Build history of the part. All positions in model axes, mm. Face numbers are marked on the shaded views. A direction names the side the tool comes from. Round coordinates to 2 decimals unless told otherwise and drop trailing zeros. Loops run counter-clockwise (first coordinate to the right, second up) from the corner with the lowest first, then second, coordinate; pieces in that order, holes last. Notation, with made-up numbers: (20.25, 11.5) - (76.25, 11.5) arc R24 ccw to (76.25, 43.5) - close; hole circle Ø10 at (24.5, 80.25). An arc over 180 degrees is marked (long way). Answer as CSV lines item,"result". Start each with the question number.
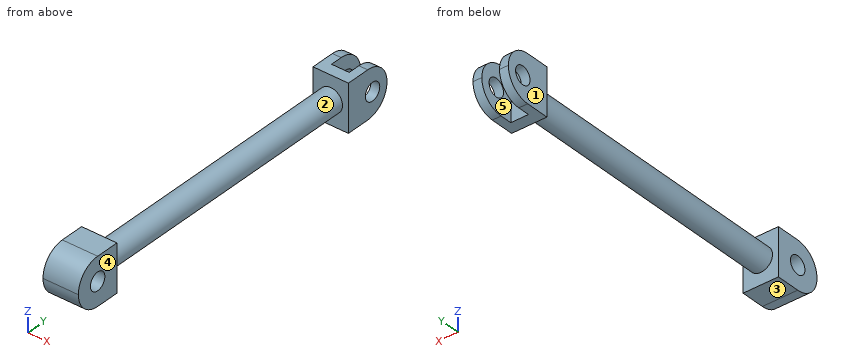
```python
from build123d import *

# Parameters (mm, degrees)
F0_R      = 12.7
F1_DEPTH  = 304.8
F2_W      = 38.1
F2_H      = 50.8
F3_DEPTH  = 50.8
F4_R      = 9.525
F5_DEPTH  = 38.101
F6_W      = 38.1
F6_H      = 50.8
F7_DEPTH  = 50.8
F8_W      = 19.05
F8_H      = 50.8
F9_DEPTH  = 38.1
F10_R     = 9.525
F11_DEPTH = 38.101
F12_R     = 25.39999


# Not quite as in the source:
# - a fillet or chamfer is up to 0.001 mm smaller than in the source, because OpenCascade refuses the exact size


with BuildPart() as f1:
    # F0 (on Front) → F1 (new body)
    with BuildSketch(Plane.XZ):
        Circle(F0_R)
    extrude(amount=F1_DEPTH)

    # F2 (on face) → F3 (join)
    with BuildSketch(Plane.XZ.offset(304.8)):
        Rectangle(F2_W, F2_H)
    extrude(amount=F3_DEPTH)

    # F4 (on face) → F5 (cut, through all)
    with BuildSketch(Plane(origin=(-19.05, 0, 0), x_dir=(0, -1, 0), z_dir=(-1, 0, 0))):
        with Locations((330.2, 0)):
            Circle(F4_R)
    extrude(amount=-F5_DEPTH, mode=Mode.SUBTRACT)

    # F6 (on face) → F7 (join)
    with BuildSketch(Plane(origin=(0, 0, 0), x_dir=(-1, 0, 0), z_dir=(0, 1, 0))):
        Rectangle(F6_W, F6_H)
    extrude(amount=F7_DEPTH)

    # F8 (on face) → F9 (cut)
    with BuildSketch(Plane(origin=(0, 50.8, 0), x_dir=(-1, 0, 0), z_dir=(0, 1, 0))):
        Rectangle(F8_W, F8_H)
    extrude(amount=-F9_DEPTH, mode=Mode.SUBTRACT)

    # F10 (on face) → F11 (cut, through all)
    with BuildSketch(Plane.YZ.offset(19.05)):
        with Locations((31.75, 0)):
            Circle(F10_R)
    extrude(amount=-F11_DEPTH, mode=Mode.SUBTRACT)

    # F12 (radius 25.4 in the source; OpenCascade refuses exactly that, so slightly less here)
    f12_edges = [f1.edges().sort_by_distance(p)[0] for p in [
        (14.2875, 50.8, 25.4),
        (14.2875, 50.8, -25.4),
        (-14.2875, 50.8, -25.4),
        (-14.2875, 50.8, 25.4),
        (0, -355.6, 25.4),
        (0, -355.6, -25.4),
    ]]
    fillet(f12_edges, radius=F12_R)


solid = f1.part
```
Q1. Band-saw the part on D-D, the plane z = -6. List the corners of the cut face in (x, y) (3 decimals).
Q2. Band-saw the part on C-C, the plane y = 31.75. List the corners of the cut face in (x, z) (3 decimals), then the cut area to 3 significant figures.
Q3. Two-plate mould, pull along X, no slides. Class the marked faces 3, 4 and 5: released by +X, released by -X, zero draft, split by the parting line, or undercut.
Q4. Band-saw the part on B-B, the plane z = -21. List the corners of the cut face in (x, y) (3 decimals), then the cut area to 3 significant figures.
Q5. Tool access for the marked faces 1 and 2: list every direction of +Z, -Z, +X, -X, +Y, -Y with a clear straight run to the whole face (end or side of a thin tool).
Q6. Pin check, flat tips, straight feed: pin 1 Ø21 at (x, z) = (-1, -8) entering from +Y; pin 2 Ø3 at (x, z) = (8, -5.5) entering from -Y; pin 3 Ø1 at (y, z) = (-78.5, 3.5) entering from -X; pin 4 Ø19 at (y, z) = (30, 7) entering from +X. Stop position of each tip, or through.
Q7. Wall check: probe 1 along Z at (x, y) = (4, -330); probe 2 along Y at (x, z) = (13.5, 4.5); probe 3 along X at (y, z) = (19.5, -23) (3 decimals). Give the ranges that are in metal, low to high. Write a range as [from, to].
Reported:
1,outline,"(-19.05, -354.881) - (19.05, -354.881) - (19.05, -337.598) - (-19.05, -337.598) - close; (-19.05, -322.802) - (19.05, -322.802) - (19.05, -304.8) - (11.193, -304.8) - (11.193, 0) - (19.05, 0) - (19.05, 24.352) - (9.525, 24.352) - (9.525, 12.7) - (-9.525, 12.7) - (-9.525, 24.352) - (-19.05, 24.352) - (-19.05, 0) - (-11.193, 0) - (-11.193, -304.8) - (-19.05, -304.8) - close; (-19.05, 39.148) - (-9.525, 39.148) - (-9.525, 50.081) - (-19.05, 50.081) - close; (9.525, 39.148) - (19.05, 39.148) - (19.05, 50.081) - (9.525, 50.081) - close"
2,outline,"(-19.05, -24.593) - (-9.525, -24.593) - (-9.525, -9.525) - (-19.05, -9.525) - close; (-19.05, 9.525) - (-9.525, 9.525) - (-9.525, 24.593) - (-19.05, 24.593) - close; (9.525, -24.593) - (19.05, -24.593) - (19.05, -9.525) - (9.525, -9.525) - close; (9.525, 9.525) - (19.05, 9.525) - (19.05, 24.593) - (9.525, 24.593) - close"
2,area,"574 mm2"
3,face 3,"zero draft"
3,face 4,"released by +X"
3,face 5,"undercut"
4,outline,"(-19.05, -344.488) - (19.05, -344.488) - (19.05, -304.8) - (-19.05, -304.8) - close; (-19.05, 0) - (19.05, 0) - (19.05, 39.688) - (9.525, 39.688) - (9.525, 12.7) - (-9.525, 12.7) - (-9.525, 39.688) - (-19.05, 39.688) - close"
4,area,"2,510 mm2"
5,face 1,"+Z, -Z, -X, +Y, -Y"
5,face 2,"none"
6,pin 1,"stops at y = 50.73"
6,pin 2,"stops at y = -355.28"
6,pin 3,"stops at x = -12.34"
6,pin 4,"stops at x = 19.05"
7,probe 1,"z = [-25.4, -9.52], [9.52, 25.4]"
7,probe 2,"y = [-355.2, -338.59], [-321.81, -304.8], [0, 23.36], [40.14, 50.4]"
7,probe 3,"x = [-19.05, -9.525], [9.525, 19.05]"
